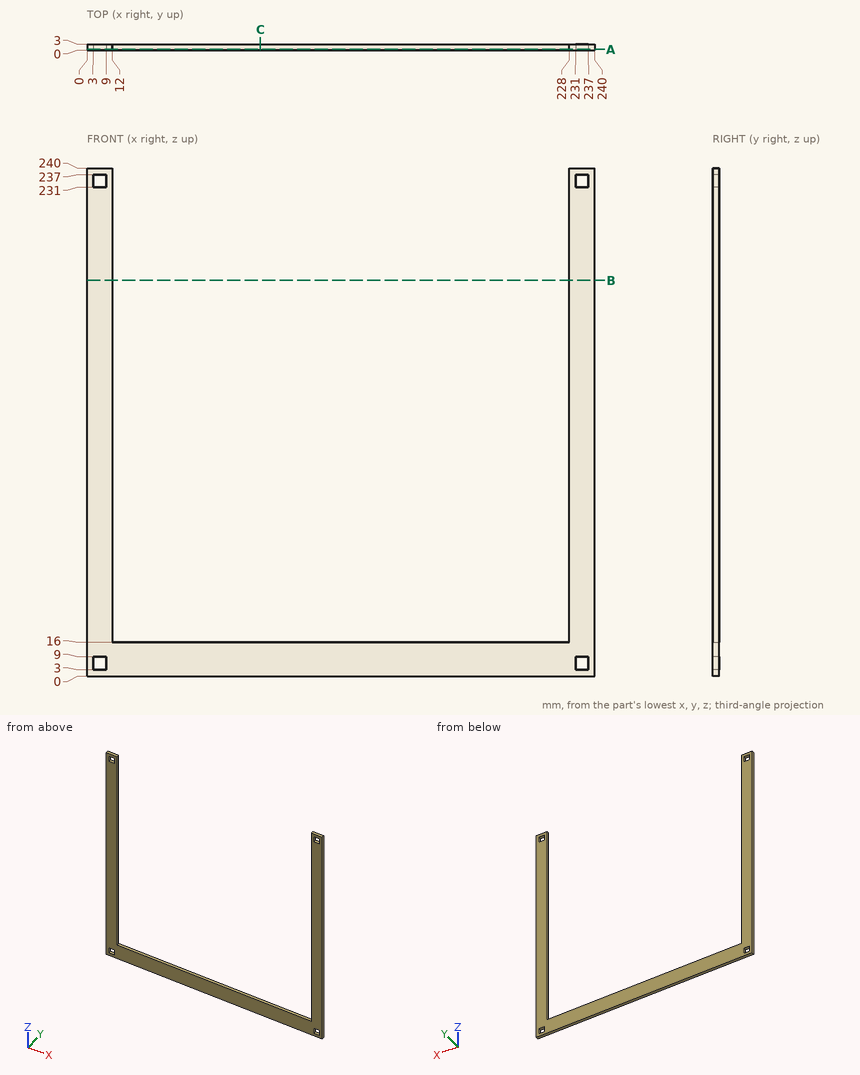
Verification items for this drawing (mm, ordinates from the low corner). Round coordinates to 2 decimals unless told otherwise and drop trailing zeros. Order: outer loops, then holes, each group sorted by start corner. A loop starts at its lowest first (then second) coordinate and runs counter-clockwise, first axis right, second up. Notation, with made-up numbers: (-10, 38.25) -> (6, 38.25) arc R12 cw to (6, 46.25) -> close; hole circle Ø3 at (-26, 17). An arc over 180 degrees is marked (long way). Use one line per item in the form item = value.
1. Cross-section at A-A, the plane y = 0.45. Enter the section's corners in (x, z).
Working result:
outline = (0, 0) -> (240, 0) -> (240, 240) -> (228, 240) -> (228, 16) -> (12, 16) -> (12, 240) -> (0, 240) -> close; hole (3, 3) -> (9, 3) -> (9, 9) -> (3, 9) -> close; hole (3, 231) -> (9, 231) -> (9, 237) -> (3, 237) -> close; hole (231, 3) -> (237, 3) -> (237, 9) -> (231, 9) -> close; hole (231, 231) -> (237, 231) -> (237, 237) -> (231, 237) -> close
2. Cross-section at C-C, the plane x = 82. Enter the section's corners in (y, z).
Working result:
outline = (0, 0) -> (3, 0) -> (3, 16) -> (0, 16) -> close
3. Go/stop test with flat-tipped pins: pin 1 (0.9 mm diameter, centred on x = 7.5, y = 1, fed in from -Z); pin 2 (0.9 mm diameter, centred on x = 142.5, y = 1, fed in from +Z). Record where each tip stops, or that it passes through.
Working result:
pin_1 = 0
pin_2 = 16
4. Cross-section at B-B, the plane z = 187. Enter the section's corners in (x, y), plus the area to 3 significant figures.
Working result:
outline = (0, 0) -> (12, 0) -> (12, 3) -> (0, 3) -> close; (228, 0) -> (240, 0) -> (240, 3) -> (228, 3) -> close
area = 72.0 mm^2
5. Scan lines: line 1 along X through (y, z) = (1.25, 158); line 2 along Z through (x, y) = (210, 1.55). Record each from-to range of solid material in increasing order. Write a range as from..to.
Working result:
line_1 = 0..12, 228..240
line_2 = 0..16
